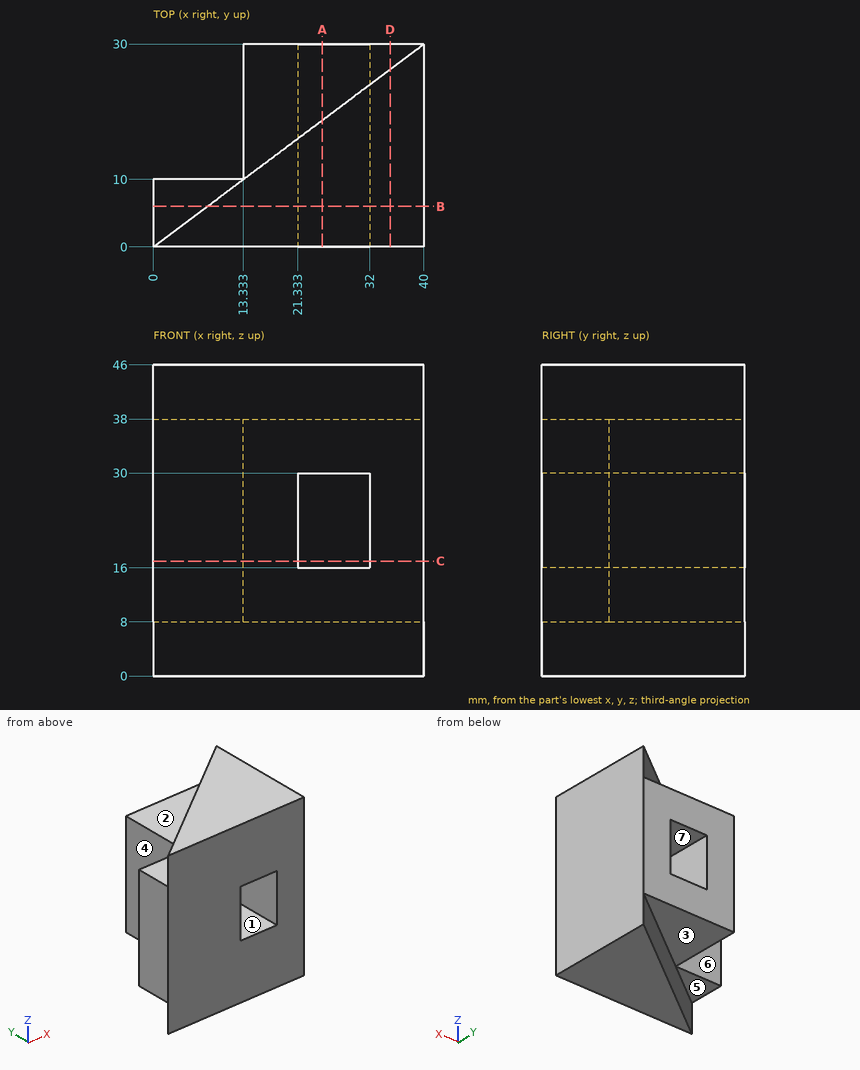
Drawing for the job (mm, zero at the part's lowest x, y, z). A direction names the side the tool comes from. Give positions to 0.01 mm unless a question says otherwise; leave off trailing zeros. Order: outer loops, then holes, each group sorted by start corner. A loop starts at its lowest first (then second) coordinate and runs counter-clockwise, first axis right, second up. Notation, with made-up numbers: M 53.25,5 L 81.25,5 A32 cw 81.25,43 Z; hole C -1.75,54 d8. An arc over 180 degrees is marked long. Put each result on its own line as item: value. Start each with the question number.
(1) Mould opens along Z. For the marked faces 5, 6 and 7 say: +Z half, -Z half, draft (parallel to the pull), parting line (faces both ways), or undercut.
(2) Saw through at C-C, the plane z = 17. Write the cut outline in (x, y), then the cut area to 3 significant figures.
(3) Saw through at B-B, the plane y = 6. Write the cut outline in (x, z), then the cut area to 3 significant figures.
(4) Flat gauge pins, fed straight in: pin 1 Ø10 at (y, z) = (17.5, 28) entering from -X; pin 2 Ø4 at (x, z) = (9, 26.5) entering from +Y; pin 3 Ø8 at (x, y) = (10.5, 25.5) entering from +Z. Where does each tip first touch, or does it go through?
(5) Saw through at D-D, the plane x = 35. Write the cut outline in (y, z).
(6) Which spindle directions (+Z, -Z, +X, -X, +Y, -Y) get a long thin tool onto all of the face, cutting with end or side? Do the marked faces 1, 2, 3 and 4. Say none if no direction does.
(7) Saw through at A-A, the plane x = 25. Write the cut outline in (y, z).
(8) Drill centre lines: line 1 along X through (y, z) = (14.5, 25.5); line 2 along Z through (x, y) = (25, 12.25); line 3 along X through (y, z) = (6.5, 25). Where is each one in solid material? Low to high.
Check result:
1. face 5: -Z half
1. face 6: draft
1. face 7: undercut
2. outline: M 0,0 L 21.33,0 L 21.33,30 L 13.33,30 L 13.33,10 L 0,10 Z; M 32,0 L 40,0 L 40,30 L 32,30 Z
2. area: 613 mm2
3. outline: M 0,8 L 8,8 L 8,0 L 40,0 L 40,46 L 8,46 L 8,38 L 0,38 Z; hole M 21.33,16 L 32,16 L 32,30 L 21.33,30 Z
3. area: 1,560 mm2
4. pin 1: stops at x = 13.33
4. pin 2: stops at y = 10
4. pin 3: stops at z = 38
5. outline: M 0,0 L 26.25,0 L 26.25,8 L 30,8 L 30,38 L 26.25,38 L 26.25,46 L 0,46 Z
6. face 1: +Y, -Y
6. face 2: +Z, -X, +Y
6. face 3: -Z, -X, +Y
6. face 4: +Z, -Z, -X, +Y
7. outline: M 0,0 L 18.75,0 L 18.75,8 L 30,8 L 30,16 L 0,16 Z; M 0,30 L 30,30 L 30,38 L 18.75,38 L 18.75,46 L 0,46 Z
8. line 1: x = 13.33 to 21.33, 32 to 40
8. line 2: z = 0 to 16, 30 to 46
8. line 3: x = 0 to 21.33, 32 to 40
